Could you check a few things on this model? Use its own coordinates, in mm. Coordinates: 2 decimals unless noted, no trailing zeros. Loops run counter-clockwise (first coordinate to the right, second up) from the corner with the lowest first, then second, coordinate; pieces in that order, holes last.
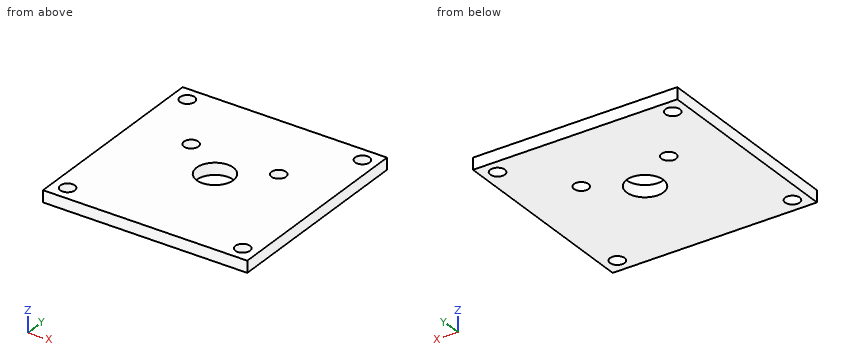
from build123d import *

# Parameters (mm, degrees)
SKETCH1_W           = 88.9
SKETCH1_H           = 88.9
BOSS_EXTRUDE1_DEPTH = 2.54
SKETCH2_R           = 3.175
SKETCH2_R_2         = 8.001
CUT_EXTRUDE1_DEPTH  = 6.08


with BuildPart() as part:
    # Sketch1 → Boss-Extrude1 (new body, symmetric)
    with BuildSketch(Plane.XY):
        with Locations((44.45, 44.45)):
            Rectangle(SKETCH1_W, SKETCH1_H)
    extrude(amount=BOSS_EXTRUDE1_DEPTH, both=True)

    # Sketch2 → Cut-Extrude1 (cut, through all)
    with BuildSketch(Plane.XY.offset(2.54)):
        with Locations((6.35, 82.55)):
            Circle(SKETCH2_R)
        with Locations((82.55, 82.55)):
            Circle(SKETCH2_R)
        with Locations((82.55, 6.35)):
            Circle(SKETCH2_R)
        with Locations((6.35, 6.35)):
            Circle(SKETCH2_R)
        with Locations((44.45, 44.45)):
            Circle(SKETCH2_R_2)
        with Locations((25.4, 57.15)):
            Circle(SKETCH2_R)
        with Locations((63.5, 57.15)):
            Circle(SKETCH2_R)
    extrude(amount=-CUT_EXTRUDE1_DEPTH, mode=Mode.SUBTRACT)


solid = part.part
1) If I drill on L1, parallel to Y at x = 6.35, z = -1 (3 decimals); L2, parallel to Y at x = 25.4, z = -0.6 (3 decimals); L3, parallel to X at y = 59.5, z = 1.45, over which ranges is the centre line in solid material (lowest first)?
2) Imagine slicing it at B-B on x = 6.35. List the corners of the cut face in (y, z) for me (3 decimals), plus the area to 3 significant figures.
3) Imagine slicing it at C-C on z = -1.4. List the corners of the cut face in (x, y) for me (3 decimals).
4) Will these pins go through, and if not, where does the flat tip stop? pin 1 (8.5 mm diameter, centred on x = 6.35, y = 82.55, fed in from +Z); pin 2 (4 mm diameter, centred on x = 25.4, y = 57.15, fed in from +Z).
5) Imagine slicing it at A-A on y = 44.45. List the corners of the cut face in (x, z) for me.
Solved:
1. L1: y = 0 to 3.175, 9.525 to 79.375, 85.725 to 88.9
1. L2: y = 0 to 53.975, 60.325 to 88.9
1. L3: x = 0 to 23.27, 27.53 to 61.37, 65.63 to 88.9
2. outline: (0, -2.54) - (3.175, -2.54) - (3.175, 2.54) - (0, 2.54) - close; (9.525, -2.54) - (79.375, -2.54) - (79.375, 2.54) - (9.525, 2.54) - close; (85.725, -2.54) - (88.9, -2.54) - (88.9, 2.54) - (85.725, 2.54) - close
2. area: 387 mm2
3. outline: (0, 0) - (88.9, 0) - (88.9, 88.9) - (0, 88.9) - close; hole circle Ø6.35 at (6.35, 6.35); hole circle Ø6.35 at (6.35, 82.55); hole circle Ø6.35 at (25.4, 57.15); hole circle Ø16.002 at (44.45, 44.45); hole circle Ø6.35 at (63.5, 57.15); hole circle Ø6.35 at (82.55, 6.35); hole circle Ø6.35 at (82.55, 82.55)
4. pin 1: stops at z = 2.54
4. pin 2: passes through
5. outline: (0, -2.54) - (36.45, -2.54) - (36.45, 2.54) - (0, 2.54) - close; (52.45, -2.54) - (88.9, -2.54) - (88.9, 2.54) - (52.45, 2.54) - close
